CAD build for the part. Positions are in the model's coordinates, mm. A direction names the side the tool comes from. Round coordinates to 2 decimals unless told otherwise and drop trailing zeros. Write each loop counter-clockwise with the first axis right and the second up, starting at its lowest first coordinate (ties: lowest second). Pieces come first, ordered by that corner, then holes. Notation, with made-up numbers: (-33.75, 15.5) - (-2.75, 15.5) arc R33 ccw to (-2.75, 50.5) - close; hole circle Ø8 at (79.25, 14). An arc over 180 degrees is marked (long way). Answer in a Markdown table with one row per item.
```python
from build123d import *
from OCP.BRepAlgoAPI import BRepAlgoAPI_Cut
from OCP.TopTools import TopTools_ListOfShape

# Parameters (mm, degrees)
CUT_EXTRUDE2_DEPTH      = 17.000000000000007
CUT_EXTRUDE2_DEPTH_BACK = 17.000000000000004
SKETCH4_R               = 1.9934980389772232
CUT_EXTRUDE3_DEPTH      = 5.000000000000005
CHAMFER1_SIZE           = 1


with BuildPart() as part:
    # Sketch1 → Revolve1 (revolve)
    with BuildSketch(Plane(origin=(0, 0, 0), x_dir=(1, 0, 0), z_dir=(0, 1, 0))):
        with BuildLine():
            Line((0, 0), (0, 38))
            Line((0, 38), (0, 53))
            ThreePointArc((0, 53), (10.60660171779814, 48.60660171779814), (15, 38))
            Line((15, 38), (10.60660171779814, 38))
            Line((10.60660171779814, 38), (10.606601717798139, -3.47e-15))
            Line((10.606601717798139, -3.47e-15), (0, 0))
        make_face()
    revolve(axis=Axis((0, 0, 0), (0, 0, -1)))


with BuildPart() as cut_extrude2_tool:
    # Sketch3 → Cut-Extrude2 (new, two sides: drawn at the far end of the back side and taken through both)
    with BuildSketch(Plane(origin=(0, 0, 0), x_dir=(1, 0, 0), z_dir=(0, 1, 0)).offset(-CUT_EXTRUDE2_DEPTH_BACK)):
        Polygon((-2.0023692524081933, 52.866942038246904), (1.9934980389762682, 52.866942038246904), (1.9934980389762682, 41), (-2.0023692524081937, 41), align=None)
    extrude(amount=CUT_EXTRUDE2_DEPTH + CUT_EXTRUDE2_DEPTH_BACK)


with BuildPart() as part_1:
    add(part.part)

    # Cut-Extrude2: cut by cut_extrude2_tool, with a tolerance
    cut_extrude2_stock = TopTools_ListOfShape()
    cut_extrude2_stock.Append(part_1.part.wrapped)
    cut_extrude2_tools = TopTools_ListOfShape()
    cut_extrude2_tools.Append(cut_extrude2_tool.part.wrapped)
    cut_extrude2_cut = BRepAlgoAPI_Cut()
    cut_extrude2_cut.SetArguments(cut_extrude2_stock)
    cut_extrude2_cut.SetTools(cut_extrude2_tools)
    cut_extrude2_cut.SetFuzzyValue(0.00001)
    cut_extrude2_cut.Build()
    add(Compound.cast(cut_extrude2_cut.Shape()).solids(), mode=Mode.REPLACE)


with BuildPart() as cut_extrude2_piece_1:
    # of the separate pieces the step leaves, piece 1, a body of its own (cut_extrude2_pieces)
    add(part_1.part.solids().sort_by_distance((1.993498039, 14.561111413, -41))[0])

    # Chamfer1
    chamfer1_edges = [cut_extrude2_piece_1.edges().sort_by_distance(p)[0] for p in [
        (-10.606601717798139, -1.3e-15, 3.47e-15),
    ]]
    chamfer(chamfer1_edges, length=CHAMFER1_SIZE)


with BuildPart() as cut_extrude2_piece_2:
    # of the separate pieces the step leaves, piece 2, a body of its own (cut_extrude2_pieces)
    add(part_1.part.solids().sort_by_distance((0, 0, -53))[0])

    # Sketch4 → Cut-Extrude3 (cut)
    with BuildSketch(Plane.XY.offset(-52.866942038246904)):
        Circle(SKETCH4_R)
    extrude(amount=-CUT_EXTRUDE3_DEPTH, mode=Mode.SUBTRACT)


solid = cut_extrude2_piece_1.part
```
Q1. Saw through at B-B on y = 0. List the corners of the cut face in (x, z).
Computed:
| item | result |
|---|---|
| outline | (-15, -38) arc R15 ccw to (-2, -52.87) - (-2, -41) - (1.99, -41) - (1.99, -52.87) arc R15 ccw to (15, -38) - (10.61, -38) - (10.61, -1) - (9.61, 0) - (-9.61, 0) - (-10.61, -1) - (-10.61, -38) - close |
Q2. Flat gauge pins, fed straight in: pin 1 (3 mm diameter, centred on x = 3, y = -9, fed in from -Z); pin 2 (2 mm diameter, centred on x = -2, y = -4, fed in from -Z); pin 3 (4 mm diameter, centred on y = 6.5, z = -30.5, fed in from -X). Where does each tip first touch, or does it go through?
Computed:
| item | result |
|---|---|
| pin 1 | stops at z = -50.7 |
| pin 2 | stops at z = -52.56 |
| pin 3 | stops at x = -9.6 |
Q3. 3-axis set-ups, long thin cutter, end or side, ignore diameter. For faces 4 (the flat face through (-4, -10, -38)), 5 (the flat face through (0, 0, -41)): which of +Z, -Z, +X, -X, +Y, -Y reach the whole face in a straight line?
Computed:
| item | result |
|---|---|
| face 4 | +Z |
| face 5 | -Z, +Y, -Y |
Q4. Saw through at A-A on x = 0. List the corners of the cut face in (y, z), then the cut area to 4 significant figures.
Computed:
| item | result |
|---|---|
| outline | (-15, -38) arc R15 ccw to (-14.7, -41) - (14.7, -41) arc R15 ccw to (15, -38) - (10.61, -38) - (10.61, -1) - (9.61, 0) - (-9.61, 0) - (-10.61, -1) - (-10.61, -38) - close |
| area | 894.5 mm2 |
Q5. Saw through at C-C on z = -18. List the corners of the cut face in (x, y), then the cut area to 3 significant figures.
Computed:
| item | result |
|---|---|
| outline | circle Ø21.21 at (0, 0) |
| area | 353 mm2 |
Q6. Pull direction X, two halves, no side cores. Call faces 1 (the flat face through (0, 0, 0)), 2 (the cylindrical face through (-8.42, 6.45, -19.24)), 3 (the flat face through (1.993, 0, -46)): released by +X, released by -X, zero draft, split by the parting line, or undercut.
Computed:
| item | result |
|---|---|
| face 1 | zero draft |
| face 2 | split by the parting line |
| face 3 | undercut |
Q7. Saw through at D-D on z = -42. List the corners of the cut face in (x, y).
Computed:
| item | result |
|---|---|
| outline | (-2, -14.32) - (-2, 14.32) arc R14.46 ccw to start; (1.99, -14.32) arc R14.46 ccw to (1.99, 14.32) - close |
Q8. Drill centre lines: line 1 (Y direction, x = -0.5, z = -19.5); line 2 (Y direction, x = 4.5, z = -25.5); line 3 (X direction, y = 0, z = -24.5). Where is each one in solid material? Low to high.
Computed:
| item | result |
|---|---|
| line 1 | y = -10.59 to 10.59 |
| line 2 | y = -9.6 to 9.6 |
| line 3 | x = -10.61 to 10.61 |
